from build123d import *

# Parameters (mm, degrees)
F0_R     = 8
F1_DEPTH = 63.15
F2_R     = 16.5
F3_DEPTH = 20
F4_R     = 16.5
F5_DEPTH = 20
F6_R     = 13.7
F6_R_2   = 7.89
F7_DEPTH = 3.75


with BuildPart() as f1:
    # F0 (on Top) → F1 (new body)
    with BuildSketch(Plane.XY):
        Polygon((32.348781, 36.45), (-32.348781, 36.45), (-36.45, 32.348781), (-36.45, 28.948781), (-30.15, 22.648781), (-27.75, 22.648781), (-27.75, 12.248781), (-36.45, 12.248781), (-36.45, -12.248781), (-27.75, -12.248781), (-27.75, -22.648781), (-30.15, -22.648781), (-36.45, -28.948781), (-36.45, -32.348781), (-32.348781, -36.45), (-28.948781, -36.45), (-22.648781, -30.15), (-22.648781, -27.75), (-12.248781, -27.75), (-12.248781, -36.45), (12.248781, -36.45), (12.248781, -27.75), (22.648781, -27.75), (22.648781, -30.15), (28.948781, -36.45), (32.348781, -36.45), (36.45, -32.348781), (36.45, 32.348781), align=None)
        Circle(F0_R, mode=Mode.SUBTRACT)
    extrude(amount=F1_DEPTH)

    # F2 (on face) → F3 (cut)
    with BuildSketch(Plane.XZ.offset(36.45)):
        with Locations((0, 31.575)):
            Circle(F2_R)
    extrude(amount=-F3_DEPTH, mode=Mode.SUBTRACT)

    # F4 (on face) → F5 (cut)
    with BuildSketch(Plane(origin=(-36.45, 0, 0), x_dir=(0, -1, 0), z_dir=(-1, 0, 0))):
        with Locations((0, 31.575)):
            Circle(F4_R)
    extrude(amount=-F5_DEPTH, mode=Mode.SUBTRACT)

    # F6 (on face) → F7 (join)
    with BuildSketch(Plane.XY.offset(63.15)):
        Circle(F6_R)
        Circle(F6_R_2, mode=Mode.SUBTRACT)
    extrude(amount=F7_DEPTH)


solid = f1.part
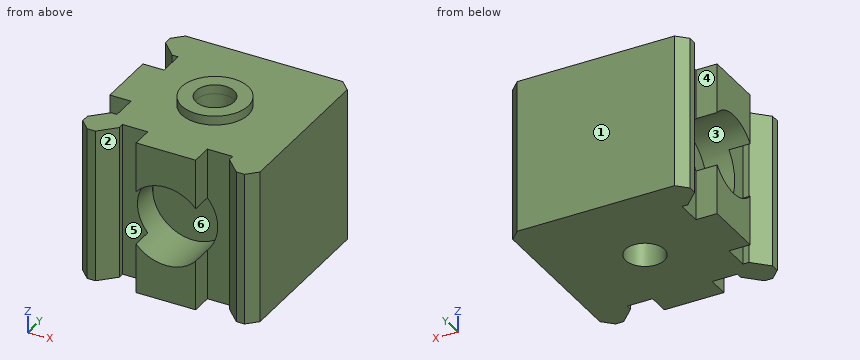
Read the model definition and answer for the solid it produces. Units are mm, in the model's axes. Face numbers are marked on the shaded views. A direction names the side the tool comes from. Give positions to 0.01 mm unless a question says otherwise; leave off trailing zeros. Loops run counter-clockwise (first coordinate to the right, second up) from the corner with the lowest first, then second, coordinate; pieces in that order, holes last. Notation, with made-up numbers: (-27, 88) -> (31, 88) arc R6 cw to (31, 98) -> close; hole circle Ø11 at (-23.75, -32). An arc over 180 degrees is marked (long way). Use a Markdown table: item, result.
Q1. Determine the mould class of the marked faces 1, 2 and 3 for opening direction Y: pulls with the +Y half, pulls with the -Y half, needs draft (parallel to the pull), parting line crosses it, or undercut.
Solved:
| item | result |
|---|---|
| face 1 | pulls with the +Y half |
| face 2 | pulls with the -Y half |
| face 3 | undercut |
Q2. A tool of negligible diameter and unlimited length cuts with its end or side. For the marked faces 4, 5 and 6, from which of +Z, -Z, +X, -X, +Y, -Y can it reach the whole face along a straight path? Write none if from no direction.
Solved:
| item | result |
|---|---|
| face 4 | +Z, -Z, -X |
| face 5 | +Z, -Z, -Y |
| face 6 | -Y |
Q3. Section D-D, the plane y = -11 is taken. Determine the outline of the cut face in (x, z).
Solved:
| item | result |
|---|---|
| outline | (-36.45, 0) -> (36.45, 0) -> (36.45, 63.15) -> (8.17, 63.15) -> (8.17, 66.9) -> (-8.17, 66.9) -> (-8.17, 63.15) -> (-36.45, 63.15) -> (-36.45, 43.87) -> (-16.45, 43.87) -> (-16.45, 19.28) -> (-36.45, 19.28) -> close |
Q4. Section A-A, the plane y = 0 is taken. Determine the outline of the cut face in (x, z) (3 decimals).
Solved:
| item | result |
|---|---|
| outline | (-36.45, 0) -> (-8, 0) -> (-8, 63.15) -> (-7.89, 63.15) -> (-7.89, 66.9) -> (-13.7, 66.9) -> (-13.7, 63.15) -> (-36.45, 63.15) -> (-36.45, 48.075) -> (-16.45, 48.075) -> (-16.45, 15.075) -> (-36.45, 15.075) -> close; (7.89, 63.15) -> (8, 63.15) -> (8, 0) -> (36.45, 0) -> (36.45, 63.15) -> (13.7, 63.15) -> (13.7, 66.9) -> (7.89, 66.9) -> close |
Q5. Find the intervals of material crossed by line 1 along Y through (x, z) = (0, 38.5); line 2 along Z through (x, y) = (0, -24) (3 decimals); line 3 along Y through (x, z) = (0, 64), in increasing order.
Solved:
| item | result |
|---|---|
| line 1 | y = -16.45 to -8, 8 to 36.45 |
| line 2 | z = 0 to 15.075, 48.075 to 63.15 |
| line 3 | y = -13.7 to -7.89, 7.89 to 13.7 |
Q6. Each of these flat-tipped pins is pushed along its axis until it touches: pin 1 (8 mm diameter, centred on x = 3, y = -1.5, fed in from -Z); pin 2 (10 mm diameter, centred on x = 5.5, z = 28, fed in from -Y); pin 3 (5 mm diameter, centred on x = 20, z = 26.5, fed in from -Y). Where does it stop, or does it pass through?
Solved:
| item | result |
|---|---|
| pin 1 | passes through |
| pin 2 | stops at y = -16.45 |
| pin 3 | stops at y = -27.75 |
